from build123d import *

# Parameters (mm, degrees)
F1_DEPTH = 150
F2_R     = 20
F3_DEPTH = 300


with BuildPart() as f1:
    # F0 (on Front) → F1 (new body, symmetric)
    with BuildSketch(Plane.XZ):
        Polygon((150, 400), (-150, 400), (-150, 350), (-130, 350), (150, 350), align=None)
    extrude(amount=F1_DEPTH, both=True)

    # F2 (on face) → F3 (join)
    with BuildSketch(Plane(origin=(0, 0, 350), x_dir=(1, 0, 0), z_dir=(0, 0, -1))):
        with Locations((110, 110)):
            Circle(F2_R)
        with Locations((-110, 110)):
            Circle(F2_R)
        with Locations((-110, -110)):
            Circle(F2_R)
        with Locations((110, -110)):
            Circle(F2_R)
    extrude(amount=F3_DEPTH)


solid = f1.part
The model under review builds one solid part; all positions refer to its coordinate system, in mm. A direction names the side the tool comes from. Round coordinates to 2 decimals unless told otherwise and drop trailing zeros. Write each loop counter-clockwise with the first axis right and the second up, starting at its lowest first coordinate (ties: lowest second). Pieces come first, ordered by that corner, then holes. Notation, with made-up numbers: M -15,-4 L 28,-4 A26 cw 28,17 Z; hole C 35,-15.5 d4. An arc over 180 degrees is marked long. Answer as CSV lines item,"result". Start each with the question number.
Q1. Tool access review of faces 4 (the face through (-2, 150, 375)), 5 (the face through (94, 122, 202)): name each direction out of +Z, -Z, +X, -X, +Y, -Y from which nothing blocks a thin tool from reaching the whole face with its end or side.
Q2. Wall thickness on line 1 along Z through (x, y) = (-67, 51); line 2 along X through (y, z) = (-100.5, 319); line 3 along Y through (x, z) = (105.5, 205.5): over which ranges is each line inside the solid? List them lowest first.
Q3. The part is to be moulded in two halves that separate along X. For faces 1 (the face through (-110, 110, 50)), 2 (the face through (-2, -2, 350)), 3 (the face through (150, -2, 375)), say which applies: +X half, -X half, draft (parallel to the pull), parting line (faces both ways), or undercut.
Q4. Consider section D-D, the plane x = -80. Give the boundary of the cut face in (y, z).
Q5. Consider section C-C, the plane z = 111. Give the boundary of the cut face in (x, y), then the cut area to 3 significant figures.
Q6. Consider section B-B, the plane y = 110. Give the boundary of the cut face in (x, z).
Q7. Consider section A-A, the plane x = -120.5. Give the boundary of the cut face in (y, z).
Q8. Clearance check with flat-ended pins moving along their axes: P1, Ø8, axis at x = 99.5, y = 53, coming from the -Z side; P2, Ø5, axis at y = 117, z = 205.5, coming from the -X side; P3, Ø6, axis at x = -117, z = 326, coming from the -Y side. State where each tip first meets the part, or that it passes through.
Result set:
1,face 4,"+Z, -Z, +X, -X, +Y"
1,face 5,"-Z"
2,line 1,"z = 350 to 400"
2,line 2,"x = -127.6 to -92.4, 92.4 to 127.6"
2,line 3,"y = -129.49 to -90.51, 90.51 to 129.49"
3,face 1,"draft"
3,face 2,"undercut"
3,face 3,"+X half"
4,outline,"M -150,350 L 150,350 L 150,400 L -150,400 Z"
5,outline,"C -110,-110 d40; C -110,110 d40; C 110,-110 d40; C 110,110 d40"
5,area,"5,030 mm²"
6,outline,"M -150,350 L -130,350 L -130,50 L -90,50 L -90,350 L 90,350 L 90,50 L 130,50 L 130,350 L 150,350 L 150,400 L -150,400 Z"
7,outline,"M -150,350 L -127.02,350 L -127.02,50 L -92.98,50 L -92.98,350 L 92.98,350 L 92.98,50 L 127.02,50 L 127.02,350 L 150,350 L 150,400 L -150,400 Z"
8,P1,"stops at z = 350"
8,P2,"stops at x = -129.49"
8,P3,"stops at y = -129.6"
